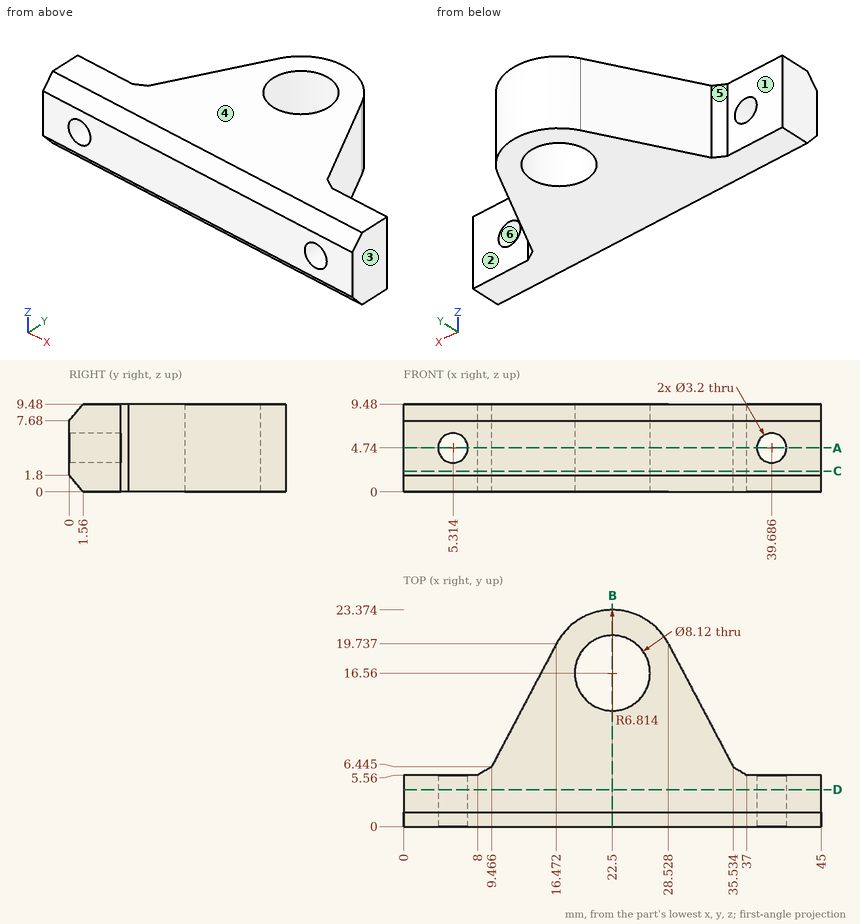
Job drawing, mm, ordinate dimensions from the low corner. One solid piece. A direction names the side the tool comes from. Round coordinates to 2 decimals unless told otherwise and drop trailing zeros. Write each loop counter-clockwise with the first axis right and the second up, starting at its lowest first coordinate (ties: lowest second). Pieces come first, ordered by that corner, then holes.
1) Mould opens along Z. For the marked faces 4, 5 and 6 say: +Z half, -Z half, draft (parallel to the pull), parting line (faces both ways), or undercut.
2) Pin check, flat tips, straight feed: pin 1 (2.5 mm diameter, centred on x = 42, z = 3.5, fed in from +Y); pin 2 (1 mm diameter, centred on x = 19.5, y = 11, fed in from -Z); pin 3 (3 mm diameter, centred on x = 37, z = 6, fed in from +Y); pin 4 (1.5 mm diameter, centred on x = 39.5, z = 1, fed in from -Y). Stop position of each tip, or through.
3) Drill centre lines: probe 1 along Y at (x, z) = (2.5, 6); probe 2 along X at (y, z) = (10.25, 4.25); probe 3 along X at (y, z) = (22.5, 4.5). Where is each one in solid material? Low to high.
4) 3-axis set-ups, long thin cutter, end or side, ignore diameter. For the marked faces 1, 2 and 3: which of +Z, -Z, +X, -X, +Y, -Y reach the whole face in a straight line?
5) Band-saw the part on A-A, the plane z = 4.74. List the corners of the cut face in (x, y) (1 decimal), and give its area (3 significant figures).
6) Band-saw the part on C-C, the plane z = 2.25. List the corners of the cut face in (x, y) (1 decimal).
7) Band-saw the part on B-B, the plane x = 22.5. List the corners of the cut face in (y, z).
8) Band-saw the part on D-D, the plane y = 4. List the corners of the cut face in (x, z).
Ans:
1. face 4: +Z half
1. face 5: draft
1. face 6: undercut
2. pin 1: stops at y = 5.56
2. pin 2: stops at z = 0
2. pin 3: stops at y = 6.51
2. pin 4: stops at y = 0.04
3. probe 1: y = 0 to 5.56
3. probe 2: x = 11.47 to 33.53
3. probe 3: x = 19.16 to 25.84
4. face 1: +Z, -Z, -X, +Y
4. face 2: +Z, -Z, +X, +Y
4. face 3: +Z, -Z, +X, +Y, -Y
5. outline: (0, 0) - (3.7, 0) - (3.7, 5.6) - (0, 5.6) - close; (6.9, 0) - (38.1, 0) - (38.1, 5.6) - (37, 5.6) - (35.5, 6.4) - (28.5, 19.7) arc R6.8 ccw to (16.5, 19.7) - (9.5, 6.4) - (8, 5.6) - (6.9, 5.6) - close; (41.3, 0) - (45, 0) - (45, 5.6) - (41.3, 5.6) - close; hole circle Ø8.1 at (22.5, 16.6)
5. area: 472 mm2
6. outline: (0, 0) - (45, 0) - (45, 5.6) - (37, 5.6) - (35.5, 6.4) - (28.5, 19.7) arc R6.8 ccw to (16.5, 19.7) - (9.5, 6.4) - (8, 5.6) - (0, 5.6) - close; hole circle Ø8.1 at (22.5, 16.6)
7. outline: (0, 1.8) - (1.56, 0) - (12.5, 0) - (12.5, 9.48) - (1.56, 9.48) - (0, 7.68) - close; (20.62, 0) - (23.37, 0) - (23.37, 9.48) - (20.62, 9.48) - close
8. outline: (0, 0) - (45, 0) - (45, 9.48) - (0, 9.48) - close; hole circle Ø3.2 at (5.31, 4.74); hole circle Ø3.2 at (39.69, 4.74)
